Check sheet for the modelled part. Datum: model origin and axes. Units: mm. Give positions to 0.01 mm unless a question says otherwise; leave off trailing zeros. Write each loop counter-clockwise with the first axis right and the second up, starting at its lowest first coordinate (ties: lowest second). Pieces come first, ordered by that corner, then holes. Notation, with made-up numbers: (16, 24) -> (39, 24) arc R13 ccw to (39, 49) -> close; hole circle Ø6 at (72.5, 27.5). An arc over 180 degrees is marked (long way). Return JSON: item names as keys, results as strings.
from build123d import *

# Parameters (mm, degrees)
ESQUISSE1_W        = 12
ESQUISSE1_H        = 12
BOSS_EXTRU_1_DEPTH = 1100
CHANFREIN1_SIZE    = 8


with BuildPart() as part:
    # Esquisse1 → Boss.-Extru.1 (new body)
    with BuildSketch(Plane.XY):
        with Locations((6, 6)):
            Rectangle(ESQUISSE1_W, ESQUISSE1_H)
    extrude(amount=BOSS_EXTRU_1_DEPTH)

    # Chanfrein1
    chanfrein1_edges = [part.edges().sort_by_distance(p)[0] for p in [
        (0, 12, 550),
    ]]
    chamfer(chanfrein1_edges, length=CHANFREIN1_SIZE)


solid = part.part
(1) Cross-section at B-B on z = 522. Enter the section's corners in (x, y), then the cut area to 3 significant figures.
Reply:
{"outline": "(0, 0) -> (12, 0) -> (12, 12) -> (8, 12) -> (0, 4) -> close", "area": "112 mm^2"}
(2) Cross-section at A-A on y = 6. Enter the section's corners in (x, z), then the cut area to 3 significant figures.
Reply:
{"outline": "(2, 0) -> (12, 0) -> (12, 1100) -> (2, 1100) -> close", "area": "11,000 mm^2"}
(3) Cross-section at C-C on x = 4.5. Enter the section's corners in (y, z), then the cut area to 3 significant figures.
Reply:
{"outline": "(0, 0) -> (8.5, 0) -> (8.5, 1100) -> (0, 1100) -> close", "area": "9,350 mm^2"}
(4) Thickness scan on L1, parallel to X at y = 8, z = 405; L2, parallel to Y at x = 1, z = 479.5; L3, parallel to X at y = 9.25, z = 267.5. Record the ranges inside material, lowest first.
Reply:
{"L1": "4 to 12", "L2": "0 to 5", "L3": "5.25 to 12"}
(5) Depth check by flat-ended pin: pin 1 Ø2 at (x, z) = (5, 629.5) entering from +Y; pin 2 Ø2 at (y, z) = (7, 209) entering from -X. Enter the tip coordinate at first touch or a pass-through.
Reply:
{"pin 1": "y = 10", "pin 2": "x = 2"}
